Verification items for the finished model (mm, model axes). Face numbers are marked on the shaded views. Round coordinates to 2 decimals unless told otherwise and drop trailing zeros. Loops run counter-clockwise (first coordinate to the right, second up) from the corner with the lowest first, then second, coordinate; pieces in that order, holes last.
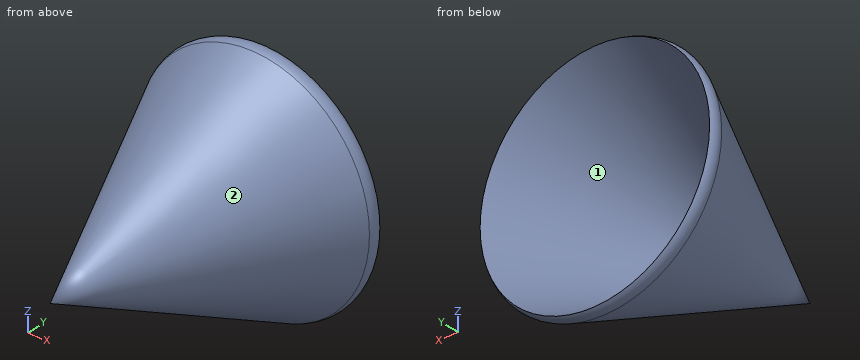
from build123d import *

# Parameters (mm, degrees)
F2_T = -2.54


# Not quite as in the source:
# - a fillet or chamfer that OpenCascade refuses, or shapes differently, is made with other operations: its cross-section is extruded or revolved along the edge and cut away or added


with BuildPart() as f1:
    # F0 (on Top) → F1 (revolve)
    with BuildSketch(Plane.XY):
        Polygon((0, 47.4987216294), (0, 44.8476299644), (0, -49.2661260068), (47.7196536958, 47.4987216294), align=None)
    revolve(axis=Axis((0, -2.2092480212, 0), (0, -1, 0)))

    # F2
    f2_openings = [f1.faces().sort_by_distance(p)[0] for p in [
        (0, 47.498722, 0),
    ]]
    offset(amount=F2_T, openings=f2_openings)

    # F3: fillet of radius 5.08 on 1 edges, made by hand

    # F3_s1 → F3_t2 (revolve, cut)
    with BuildSketch(Plane.XY):
        with BuildLine():
            ThreePointArc((45.2198112097, 42.4295968862), (45.7328319828, 45.0086691469), (44.8875848746, 47.4987216294))
            Line((44.8875848746, 47.4987216294), (47.7196536958, 47.4987216294))
            Line((47.7196536958, 47.4987216294), (45.2198112097, 42.4295968862))
        make_face()
    revolve(axis=Axis((0, 47.4987216294, 0), (0, -1, 0)), mode=Mode.SUBTRACT)


solid = f1.part
1. Section check B-B (y = 25.5). Enter the section's corners in (x, z), then the cut area to 3 significant figures.
2. Release check for a two-part mould opening along Z. For the marked faces 1 and 2 record: released by +Z, released by -Z, zero draft, split by the parting line, or undercut.
3. Section check A-A (y = 13.5). Enter the section's corners in (x, z), then the cut area to 3 significant figures.
4. Gauge pin test, flat ends, axial feed: P1, Ø1.5, axis at y = 25.5, z = 5, coming from the +X side; P2, Ø6, axis at y = 3, z = -9.5, coming from the -X side; P3, Ø4, axis at y = -2.5, z = -12.5, coming from the +X side. Record the tip position at first contact, or that the pin passes through.
5. Scan lines: L1, parallel to X at y = 2, z = -8; L2, parallel to X at y = 42, z = -3; L3, parallel to Z at x = 25.5, y = 30. Record each from-to range of solid material in increasing order.
Taken from the geometry:
1. outline: circle Ø73.74 at (0, 0); hole circle Ø68.08 at (0, 0)
1. area: 631 mm2
2. face 1: undercut
2. face 2: split by the parting line
3. outline: circle Ø61.91 at (0, 0); hole circle Ø56.24 at (0, 0)
3. area: 526 mm2
4. P1: stops at x = 36.92
4. P2: stops at x = -25.85
4. P3: stops at x = 21.02
5. L1: x = -23.98 to -20.98, 20.98 to 23.98
5. L2: x = -44.91 to -42.07, 42.07 to 44.91
5. L3: z = -29.63 to -25.78, 25.78 to 29.63
